from build123d import *

# Parameters (mm, degrees)
F0_R        = 26.1
F1_DEPTH    = 3
F2_R        = 16.3023270164
F3_DEPTH    = 1
F5_R        = 2.8
F6_DEPTH    = 3.0010001
F8_DEPTH    = 2
F9_T2_ANGLE = 247.8747937478
F9_T4_ANGLE = 287.2551612694
F11_R       = 3.5
F12_DEPTH   = 2
F14_ANGLE   = 180
F16_R       = 26.1
F16_R_2     = 2.8
F17_DEPTH   = 1


# Not quite as in the source:
# - a fillet or chamfer that OpenCascade refuses, or shapes differently, is made with other operations: its cross-section is extruded or revolved along the edge and cut away or added


with BuildPart() as f1:
    # F0 (on Top) → F1 (new body)
    with BuildSketch(Plane.XY):
        Circle(F0_R)
    extrude(amount=F1_DEPTH)

    # F2 (on face) → F3 (cut)
    with BuildSketch(Plane.XY.offset(3)):
        Circle(F2_R)
    extrude(amount=-F3_DEPTH, mode=Mode.SUBTRACT)

    # F4: fillet of radius 5 on 2 edges, made by hand

    # F4_s1 → F4_t2 (revolve, cut)
    with BuildSketch(Plane.XZ):
        with BuildLine():
            ThreePointArc((26.1, 0), (24.2560370926, 2.1833001327), (21.517424305, 3))
            Line((21.517424305, 3), (26.1, 3))
            Line((26.1, 3), (26.1, 0))
        make_face()
    revolve(axis=Axis((0, 0, 3), (0, 0, 1)), mode=Mode.SUBTRACT)

    # F4_s3 → F4_t4 (revolve, cut)
    with BuildSketch(Plane.XZ):
        with BuildLine():
            ThreePointArc((19.3023270164, 3), (17.7211881863, 2.7434164903), (16.3023270164, 2))
            Line((16.3023270164, 2), (16.3023270164, 3))
            Line((16.3023270164, 3), (19.3023270164, 3))
        make_face()
    revolve(axis=Axis((0, 0, 3), (0, 0, 1)), mode=Mode.SUBTRACT)

    # F5 (on Top) → F6 (cut, through all)
    with BuildSketch(Plane.XY):
        with Locations((0, 19.75)):
            Circle(F5_R)
        with Locations((-19.75, 0)):
            Circle(F5_R)
        with Locations((0, -19.75)):
            Circle(F5_R)
        with Locations((19.75, 0)):
            Circle(F5_R)
    extrude(amount=F6_DEPTH, mode=Mode.SUBTRACT)

    # F7 (on face) → F8 (join)
    with BuildSketch(Plane.XY.offset(2)):
        with BuildLine():
            ThreePointArc((11.5, 4.8023270164), (0, -6.6976729836), (-11.5, 4.8023270164))
            ThreePointArc((-11.5, 4.8023270164), (0, -12.3023270164), (11.5, 4.8023270164))
        make_face()
    extrude(amount=F8_DEPTH)

    # F9: fillet of radius 2.85 on 2 edges, made by hand

    # F9_s1 → F9_t2 (revolve, cut)
    with BuildSketch(Plane(origin=(-2.2243490984, 3.3055181298, 0), x_dir=(0, 0, 1), z_dir=(-0.558286738, 0.8296480689, 0))):
        with BuildLine():
            ThreePointArc((2, 14.1810754847), (3.4461925006, 15.2131752848), (4, 16.9013695864))
            Line((4, 16.9013695864), (4, 14.1810754847))
            Line((4, 14.1810754847), (2, 14.1810754847))
        make_face()
    revolve(axis=Axis((0, 4.8023270164, 4), (0, 0, -1)), revolution_arc=F9_T2_ANGLE, mode=Mode.SUBTRACT)

    # F9_s3 → F9_t4 (revolve, cut)
    with BuildSketch(Plane(origin=(0.0553451509, 0.0407628561, 0), x_dir=(0, 0, 1), z_dir=(0.8051793599, 0.5930313638, 0))):
        with BuildLine():
            ThreePointArc((2, -12.5115597549), (3.4461925006, -11.4794599548), (4, -9.7912656532))
            Line((4, -9.7912656532), (4, -12.5115597549))
            Line((4, -12.5115597549), (2, -12.5115597549))
        make_face()
    revolve(axis=Axis((0, 0.1159068972, 4), (0, 0, 1)), revolution_arc=F9_T4_ANGLE, mode=Mode.SUBTRACT)

    # F11 (on offset) → F12 (cut)
    with BuildSketch(Plane.XY.offset(3)):
        with Locations((0, 19.75)):
            Circle(F11_R)
        with Locations((19.75, 0)):
            Circle(F11_R)
        with Locations((0, -19.75)):
            Circle(F11_R)
        with Locations((-19.75, 0)):
            Circle(F11_R)
    extrude(amount=-F12_DEPTH, mode=Mode.SUBTRACT)

    # F13 (on Top) → F14 (revolve)
    with BuildSketch(Plane.XY):
        with BuildLine():
            Line((0, 12.3023270164), (0, -2.6976729836))
            ThreePointArc((0, -2.6976729836), (7.5, 4.8023270164), (0, 12.3023270164))
        make_face()
    revolve(axis=Axis((0, 4.8023270164, 0), (0, -1, 0)), revolution_arc=F14_ANGLE)


with BuildPart() as f1_1:
    # F15: moved
    add(f1.part.moved(Location((0, 0, 1))))

    # F16 (on face) → F17 (join)
    with BuildSketch(Plane(origin=(0, 0, 1), x_dir=(1, 0, 0), z_dir=(0, 0, -1))):
        Circle(F16_R)
        with Locations((0, -19.75)):
            Circle(F16_R_2, mode=Mode.SUBTRACT)
        with Locations((-19.75, 0)):
            Circle(F16_R_2, mode=Mode.SUBTRACT)
        with Locations((19.75, 0)):
            Circle(F16_R_2, mode=Mode.SUBTRACT)
        with Locations((0, 19.75)):
            Circle(F16_R_2, mode=Mode.SUBTRACT)
    extrude(amount=F17_DEPTH)


solid = f1_1.part
Verification items for the finished model (mm, model axes). A direction names the side the tool comes from. Coordinates: 2 decimals unless noted, no trailing zeros. One line per item, written item: value. Start each with the question number.
Q1. Go/stop test with flat-tipped pins: P1, Ø5, axis at x = 14.5, y = 17, coming from the +Z side; P2, Ø6.5, axis at x = -19.75, y = 0, coming from the +Z side; P3, Ø1, axis at y = 19.5, z = 5, coming from the +X side; P4, Ø20, axis at x = 8.5, y = -11, coming from the +Z side. Record where each tip stops, or that it passes through.
Q2. Mould release check, pull along X, two halves, no side actions. Record for faces 1 (the cylindrical face through (-19.237, -17.64, 0.507)), 2 (the flat face through (14, -14, 4)), 3 (the cylindrical face through (-0.46, 23.22, 3.01)): pulls with the +X half, pulls with the -X half, needs draft (parallel to the pull), parting line crosses it, or undercut.
Q3. Access from +Z, -Z, +X, -X, +Y, -Y to the whole of each face (thin tool, end or side, straight path). Record for faces 4 (the cylindrical face through (-22.547, -0.123, 1.014)), 5 (the flat face through (-14, 14, 4)), 6 (the flat face through (14, 14, 4)), 7 (the flat face through (-3, -21, 2)), 8 (the flat face through (-14, -14, 4)).
Q4. Thickness scan on L1, parallel to Y at x = 0, z = 0.75; L2, parallel to X at y = -2.5, z = 1. Record the ranges inside material, lowest first. Write a range as from..to.
Checked values:
1. P1: stops at z = 4
1. P2: stops at z = 2
1. P3: passes through
1. P4: stops at z = 5
2. face 1: parting line crosses it
2. face 2: needs draft
2. face 3: undercut
3. face 4: +Z, -Z
3. face 5: +Z, -X, +Y
3. face 6: +Z, +X, +Y
3. face 7: +Z
3. face 8: +Z, -X, -Y
4. L1: y = -26.1..-22.55, -16.95..16.95, 22.55..26.1
4. L2: x = -25.98..-21.01, -18.49..18.49, 21.01..25.98
